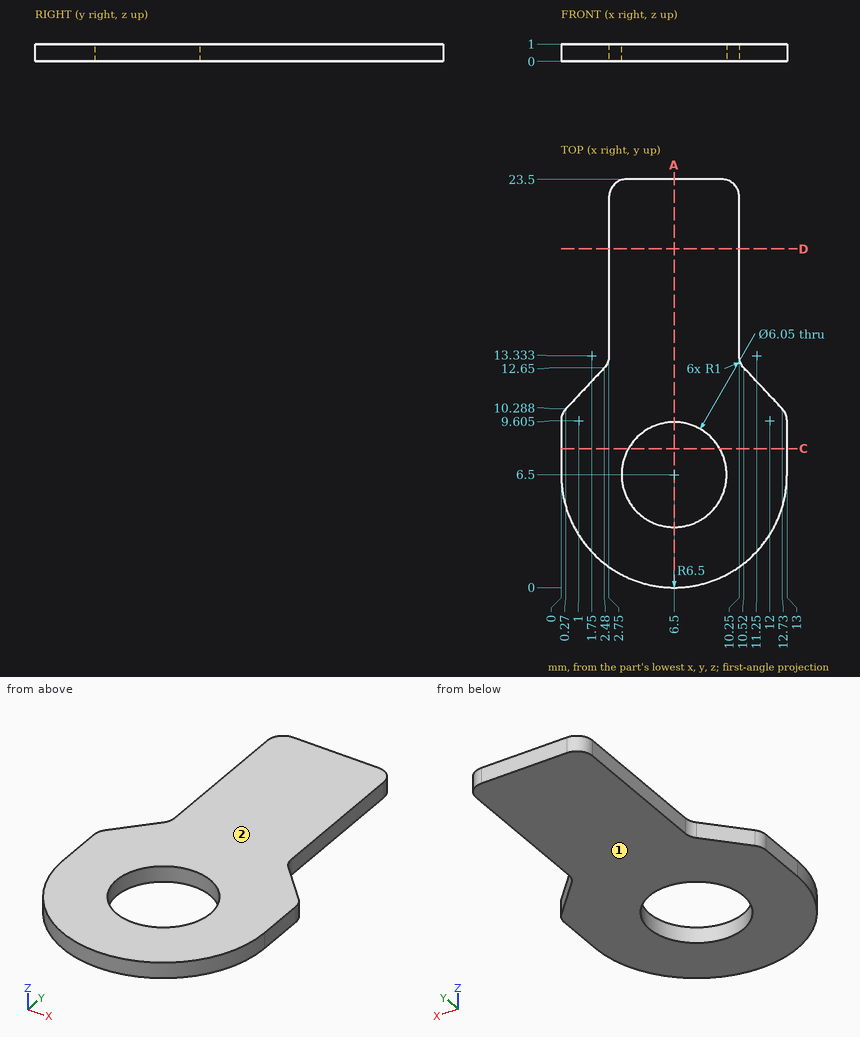
Geometry: see drawing. Coordinates: mm, zero at the bounding-box minimum. Coordinates: 2 decimals unless noted, no trailing zeros. Order: outer loops, then holes, each group sorted by start corner. A loop starts at its lowest first (then second) coordinate and runs counter-clockwise, first axis right, second up. Notation, with made-up numbers: (83, 59.25) -> (94, 59.25) arc R22 ccw to (94, 93.25) -> close; hole circle Ø2 at (59.5, 80). An arc over 180 degrees is marked (long way). Write each question's results on one line, items separated by ' | '. Start each with the question number.
1) Mould query, pull axis Z, two halves, no side actions, for the marked faces 1 and 2. Classes: released by +Z, released by -Z, zero draft, split by the parting line, or undercut.
2) First-contact query: pin 1 (5 mm diameter, centred on x = 6.5, y = 6.5, fed in from -Z). Flat tip, straight axial feed; report the tip coordinate or a pass-through.
3) Cut plane A-A, the plane x = 6.5. Output: boundary loops of the cut face in (y, z) (1 decimal).
4) Cut plane D-D, the plane y = 19.5. Output: boundary loops of the cut face in (x, z).
5) Cut plane C-C, the plane y = 8. Output: boundary loops of the cut face in (x, z).
6) Material intervals for line 1 along Y through (x, z) = (6.5, 0.4) (1 decimal); line 2 along X through (y, z) = (7.75, 0.35) (1 decimal); line 3 along X through (y, z) = (9.25, 0.15), sorted ascending.
Checks:
1) face 1: released by -Z | face 2: released by +Z
2) pin 1: through
3) outline: (0, 0) -> (3.5, 0) -> (3.5, 1) -> (0, 1) -> close; (9.5, 0) -> (23.5, 0) -> (23.5, 1) -> (9.5, 1) -> close
4) outline: (2.75, 0) -> (10.25, 0) -> (10.25, 1) -> (2.75, 1) -> close
5) outline: (0, 0) -> (3.87, 0) -> (3.87, 1) -> (0, 1) -> close; (9.13, 0) -> (13, 0) -> (13, 1) -> (9.13, 1) -> close
6) line 1: 0 to 3.5, 9.5 to 23.5 | line 2: 0 to 3.7, 9.3 to 13 | line 3: 0 to 5.24, 7.76 to 13
